```python
from build123d import *

# Parameters (mm, degrees)
SKETCH1_W           = 15
SKETCH1_H           = 15
BOSS_EXTRUDE1_DEPTH = 5
SKETCH2_R           = 4
SKETCH2_R_2         = 2.5
BOSS_EXTRUDE2_DEPTH = 3
BOSS_EXTRUDE2_DRAFT = 1
FILLET1_R           = 0.3
SKETCH3_R           = 4
BOSS_EXTRUDE3_DEPTH = 10


with BuildPart() as part:
    # Sketch1 → Boss-Extrude1 (new body)
    with BuildSketch(Plane(origin=(0, 0, 0), x_dir=(1, 0, 0), z_dir=(0, 1, 0))):
        Rectangle(SKETCH1_W, SKETCH1_H)
    extrude(amount=BOSS_EXTRUDE1_DEPTH)


with BuildPart() as boss_extrude2_tool:
    # Sketch2 → Boss-Extrude2 (with draft: the straight prism first)
    with BuildSketch(Plane(origin=(0, 5, 0), x_dir=(1, 0, 0), z_dir=(0, 1, 0))):
        Circle(SKETCH2_R)
        Circle(SKETCH2_R_2, mode=Mode.SUBTRACT)
    extrude(amount=BOSS_EXTRUDE2_DEPTH)
    # Boss-Extrude2: the draft: its side faces are tilted about the plane it starts from
    boss_extrude2_sides = [boss_extrude2_tool.faces().sort_by_distance(p)[0] for p in [
        (-4, 6.5, 0),
        (-2.5, 6.5, 0),
    ]]
    draft(boss_extrude2_sides, Plane(origin=(0, 5, 0), x_dir=(1, 0, 0), z_dir=(0, 1, 0)), BOSS_EXTRUDE2_DRAFT)


with BuildPart() as part_1:
    add(part.part)

    # Boss-Extrude2: add boss_extrude2_tool
    add(boss_extrude2_tool.part)

    # Fillet1
    fillet1_edges = [part_1.edges().sort_by_distance(p)[0] for p in [
        (-3.947634805, 8, 0),
        (-2.552365195, 8, 0),
    ]]
    fillet(fillet1_edges, radius=FILLET1_R)

    # Sketch3 → Boss-Extrude3 (add)
    with BuildSketch(Plane.XZ):
        with Locations(Location((0, 0, 0), (0, 0, 270))):
            Circle(SKETCH3_R)
    extrude(amount=BOSS_EXTRUDE3_DEPTH)


solid = part_1.part
```
Here's how the part is built. I have some questions about the finished solid (model axes, mm). A direction names the side the tool comes from. Round coordinates to 2 decimals unless told otherwise and drop trailing zeros. Order: outer loops, then holes, each group sorted by start corner. A loop starts at its lowest first (then second) coordinate and runs counter-clockwise, first axis right, second up. Notation, with made-up numbers: (49, 25) -> (65, 25) arc R22 cw to (65, 43) -> close; hole circle Ø7 at (29, -12). An arc over 180 degrees is marked (long way). Use a Markdown table: item, result. Add a question column.
(1) I need wall thicknesses on line 1 along Y through (x, z) = (3, 2.75); line 2 along X through (y, z) = (5.75, -0.25); line 3 along Y through (x, z) = (-0.75, 1). Which ranges of each line are inside material? Lowest first, please.
(2) Suppose I cut it at A-A, the plane x = -6. Please give me the cut outline in (y, z), and give its area (3 significant figures).
(3) Suppose I cut it at D-D, the plane y = -6.25. Please give me the cut outline in (x, z), and give its area (3 significant figures).
(4) If we mould it in two halves opening along Z, with no side actions, what happens to faces 4 (the face through (7.5, 2, 0)), 5 (the face through (0, 2, 7.5)), 6 (the face through (-0.547, 6.334, 2.463))? For each: released by +Z, released by -Z, zero draft, split by the parting line, or undercut.
(5) For pin 1 Ø3 at (x, z) = (5, -4.5) entering from -Y, with a flat end and sliding along its axis, tell me the tip position at first contact or that it passes through.
(6) Suppose I cut it at B-B, the plane y = 5.75. Please give me the cut outline in (x, z), and give its area (3 significant figures).
(7) For faces 1 (the face through (3.793, 6.334, -1.194)), 2 (the face through (0, 2, -7.5)), 3 (the face through (-3, 0, -3)), which set-ups out of +Z, -Z, +X, -X, +Y, -Y let a thin tool reach every point of the face, with its end or its side?
(8) Suppose I cut it at C-C, the plane z = 5.25. Please give me the cut outline in (x, y), and give its area (3 significant figures).
Verdict:
| question | item | result |
|---|---|---|
| 1 | line 1 | 0 to 5 |
| 1 | line 2 | -3.98 to -2.5, 2.5 to 3.98 |
| 1 | line 3 | -10 to 5 |
| 2 | outline | (0, -7.5) -> (5, -7.5) -> (5, 7.5) -> (0, 7.5) -> close |
| 2 | area | 75.0 mm2 |
| 3 | outline | circle Ø8 at (0, 0) |
| 3 | area | 50.3 mm2 |
| 4 | face 4 | zero draft |
| 4 | face 5 | released by +Z |
| 4 | face 6 | undercut |
| 5 | pin 1 | y = 0 |
| 6 | outline | circle Ø7.97 at (0, 0); hole circle Ø5.03 at (0, 0) |
| 6 | area | 30.1 mm2 |
| 7 | face 1 | +Y |
| 7 | face 2 | -Z, +X, -X, +Y, -Y |
| 7 | face 3 | -Y |
| 8 | outline | (-7.5, 0) -> (7.5, 0) -> (7.5, 5) -> (-7.5, 5) -> close |
| 8 | area | 75.0 mm2 |
